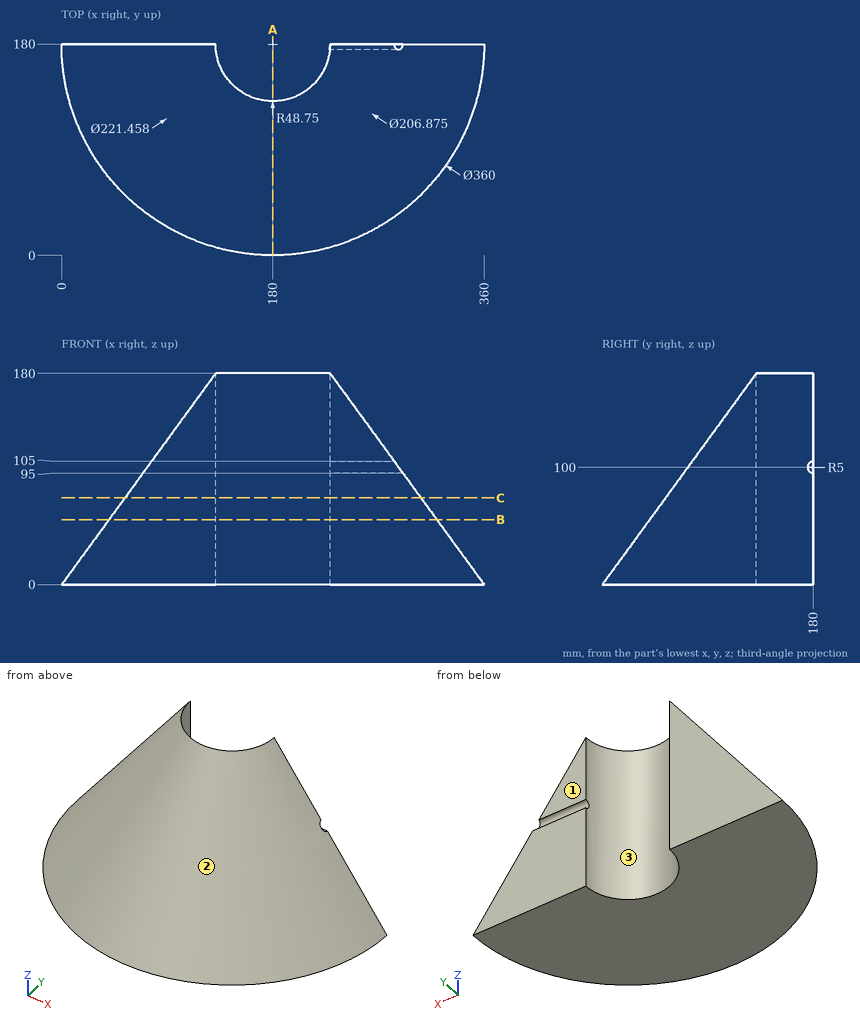
Geometry check sheet. Reference: drawing and pictorial views, mm from the part's lowest x, y, z. Give positions to 0.01 mm unless a question says otherwise; leave off trailing zeros. Write each loop counter-clockwise with the first axis right and the second up, starting at its lowest first coordinate (ties: lowest second). Pieces come first, ordered by that corner, then holes. Notation, with made-up numbers: (60, -11.75) -> (66, -11.75) arc R18 ccw to (66, 12.25) -> close; hole circle Ø9 at (-10, 70). An arc over 180 degrees is marked (long way). One line per item, written item: value. Start each with the question number.
Item 1: Gauge pin test, flat ends, axial feed: pin 1 (1 mm diameter, centred on x = 102, y = 99, fed in from +Z) (1 decimal); pin 2 (1.5 mm diameter, centred on x = 95.5, y = 101, fed in from +Z); pin 3 (6 mm diameter, centred on y = 128.5, z = 52, fed in from +X) (1 decimal). Record the tip position at first contact, or that the pin passes through.
Item 2: Draft check along X on the marked faces 1, 2 and 3. Enter one of: +X half, -X half, draft (parallel to the pull), parting line (faces both ways), or undercut.
Item 3: Section check C-C on z = 74. Record the cut outline in (x, y).
Item 4: Section check B-B on z = 55.5. Record the cut outline in (x, y).
Item 5: Section check A-A on x = 180. Record the cut outline in (y, z), then the cut area to 3 significant figures.
Item 6: Material ranges on probe 1 along X at (y, z) = (155, 48); probe 2 along X at (y, z) = (147, 45); probe 3 along Y at (x, z) = (264.5, 49.5) (1 decimal), recorded low to high. Write a range as from..to.
Results list:
1. pin 1: z = 93.3
1. pin 2: z = 89.24
1. pin 3: x = 315
2. face 1: draft
2. face 2: parting line
2. face 3: undercut
3. outline: (53.96, 180) arc R126.04 ccw to (306.04, 180) -> (228.75, 180) arc R48.75 cw to (131.25, 180) -> close
4. outline: (40.47, 180) arc R139.53 ccw to (319.53, 180) -> (228.75, 180) arc R48.75 cw to (131.25, 180) -> close
5. outline: (0, 0) -> (131.25, 0) -> (131.25, 180) -> close
5. area: 11,800 mm²
6. probe 1: 37.17..138.15, 221.85..322.83
6. probe 2: 36.56..144.12, 215.88..323.44
6. probe 3: 63.5..180
